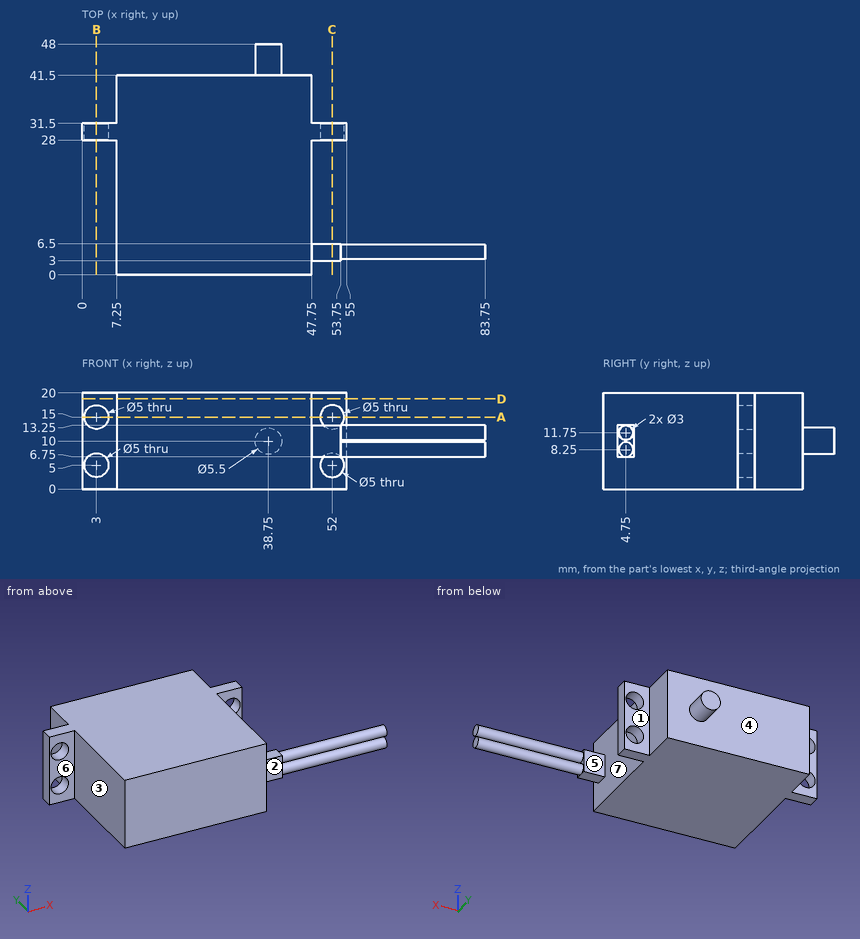
Check sheet for the drawn part. Datum: minimum x, y, z corner. Units: mm. A direction names the side the tool comes from. Coordinates: 2 decimals unless noted, no trailing zeros. Loops run counter-clockwise (first coordinate to the right, second up) from the corner with the lowest first, then second, coordinate; pieces in that order, holes last. Notation, with made-up numbers: (-9.5, -6) - (44.5, -6) arc R18 cw to (44.5, 19) - close; hole circle Ø3 at (13.5, 30.5). An arc over 180 degrees is marked (long way). Put each result on its own line as item: value.
Item 1: Section check D-D (z = 18.75). Enter the section's corners in (x, y).
Conclusion:
outline: (0, 28) - (7.25, 28) - (7.25, 0) - (47.75, 0) - (47.75, 28) - (55, 28) - (55, 31.5) - (47.75, 31.5) - (47.75, 41.5) - (7.25, 41.5) - (7.25, 31.5) - (0, 31.5) - close
Item 2: Gauge pin test, flat ends, axial feed: pin 1 Ø3.5 at (x, z) = (4, 14) entering from +Y; pin 2 Ø3 at (x, y) = (50.5, 5) entering from -Z; pin 3 Ø8 at (y, z) = (36, 6.5) entering from +X; pin 4 Ø4 at (x, z) = (3, 5) entering from -Y. Record the tip position at first contact, or that the pin passes through.
Conclusion:
pin 1: stops at y = 31.5
pin 2: stops at z = 6.75
pin 3: stops at x = 47.75
pin 4: passes through
Item 3: Section check C-C (x = 52). Enter the section's corners in (y, z), then the cut area to 4 significant figures.
Conclusion:
outline: (3, 6.75) - (6.5, 6.75) - (6.5, 13.25) - (3, 13.25) - close; (28, 0) - (31.5, 0) - (31.5, 2.5) - (28, 2.5) - close; (28, 7.5) - (31.5, 7.5) - (31.5, 12.5) - (28, 12.5) - close; (28, 17.5) - (31.5, 17.5) - (31.5, 20) - (28, 20) - close
area: 57.75 mm2
Item 4: Draft check along Y on the marked faces 4, 5, 6 and 7. Enter one of: pulls with the +Y half, pulls with the -Y half, needs draft (parallel to the pull), parting line crosses it, or undercut.
Conclusion:
face 4: pulls with the +Y half
face 5: undercut
face 6: pulls with the -Y half
face 7: undercut
Item 5: Section check A-A (z = 15). Enter the section's corners in (x, y), then the cut area to 3 significant figures.
Conclusion:
outline: (0, 28) - (0.5, 28) - (0.5, 31.5) - (0, 31.5) - close; (5.5, 28) - (7.25, 28) - (7.25, 0) - (47.75, 0) - (47.75, 28) - (49.5, 28) - (49.5, 31.5) - (47.75, 31.5) - (47.75, 41.5) - (7.25, 41.5) - (7.25, 31.5) - (5.5, 31.5) - close; (54.5, 28) - (55, 28) - (55, 31.5) - (54.5, 31.5) - close
area: 1,700 mm2
Item 6: Scan lines: line 1 along X through (y, z) = (30.7, 15); line 2 along Z through (x, y) = (52, 29); line 3 along Y through (x, z) = (35, 12.5). Record each from-to range of solid material in increasing order.
Conclusion:
line 1: x = 0 to 0.5, 5.5 to 49.5, 54.5 to 55
line 2: z = 0 to 2.5, 7.5 to 12.5, 17.5 to 20
line 3: y = 0 to 41.5
Item 7: Set-up check for the marked faces 1, 2 and 3: record each of +Z, -Z, +X, -X, +Y, -Y from which the full face is reachable in a straight line by a thin tool's end or side.
Conclusion:
face 1: +Z, -Z, +X, +Y
face 2: +Z, -Z, +X, -Y
face 3: +Z, -Z, -X, -Y
Item 8: Section check B-B (x = 3). Enter the section's corners in (y, z).
Conclusion:
outline: (28, 0) - (31.5, 0) - (31.5, 2.5) - (28, 2.5) - close; (28, 7.5) - (31.5, 7.5) - (31.5, 12.5) - (28, 12.5) - close; (28, 17.5) - (31.5, 17.5) - (31.5, 20) - (28, 20) - close
